For this review, take the finished solid that the model builds, in its own axes (mm). A direction names the side the tool comes from. Round coordinates to 2 decimals unless told otherwise and drop trailing zeros. One line per question, with ' | ' between items.
```python
from build123d import *

# Parameters (mm, degrees)
EXTRUDE_1_DEPTH = 10
SHELL_2_T       = 3
FILLET_3_R      = 10
FILLET_4_R      = 3
SKETCH_2_R      = 2.65
EXTRUDE_2_DEPTH = 8
FILLET_7_R      = 5
CHAMFER_1_SIZE  = 0.2
CHAMFER_2_SIZE  = 0.2
FILLET_9_R      = 2
FILLET_10_R     = 2


# Some blends are built 0.0001 mm under size
with BuildPart() as part:
    # 草图1 → 凸台-拉伸1 (new body)
    with BuildSketch(Plane(origin=(0, 0, 0), x_dir=(1, 0, 0), z_dir=(0, 1, 0))):
        with BuildLine():
            Line((-37.5, 15), (37.5, 15))
            ThreePointArc((37.5, 15), (44.571067812, 12.071067812), (47.5, 5))
            Line((47.5, 5), (47.5, -5))
            ThreePointArc((47.5, -5), (44.571067812, -12.071067812), (37.5, -15))
            Line((37.5, -15), (-37.5, -15))
            ThreePointArc((-37.5, -15), (-44.571067812, -12.071067812), (-47.5, -5))
            Line((-47.5, -5), (-47.5, 5))
            ThreePointArc((-47.5, 5), (-44.571067812, 12.071067812), (-37.5, 15))
        make_face()
    extrude(amount=EXTRUDE_1_DEPTH)

    # 抽壳2
    shell_2_openings = [part.faces().sort_by_distance(p)[0] for p in [
        (0, 0, 0),
    ]]
    offset(amount=SHELL_2_T, openings=shell_2_openings, kind=Kind.INTERSECTION)

    # 圆角3
    # the kernel refuses this fillet: 10 mm, written as the material it takes off along each edge
    with BuildSketch(Plane(origin=(37.5, 13, 5), x_dir=(1, 0, 0), z_dir=(0, 0, -1))) as fillet_3_piece_1:
        with BuildLine():
            CenterArc((13 - FILLET_3_R, FILLET_3_R), FILLET_3_R, 270, 90)
            Line((13 - FILLET_3_R, 0), (13, 0))
            Line((13, 0), (13, FILLET_3_R))
        make_face()
    revolve(axis=Axis((37.5, 13, 5), (0, -1, 0)), revolution_arc=90, mode=Mode.SUBTRACT)
    with BuildSketch(Plane(origin=(50.5, 13, 5), x_dir=(0, -1, 0), z_dir=(0, 0, -1)), Plane(origin=(-50.5, 13, -5), x_dir=(0, -1, 0), z_dir=(0, 0, 1))) as fillet_3_piece_2:
        with BuildLine():
            CenterArc((FILLET_3_R, FILLET_3_R), FILLET_3_R, 180, 90)
            Line((0, FILLET_3_R), (0, 0))
            Line((0, 0), (FILLET_3_R, 0))
        make_face()
    extrude(amount=10, mode=Mode.SUBTRACT)
    with BuildSketch(Plane(origin=(37.5, 13, -5), x_dir=(0, 0, -1), z_dir=(-1, 0, 0))) as fillet_3_piece_3:
        with BuildLine():
            CenterArc((13 - FILLET_3_R, FILLET_3_R), FILLET_3_R, 270, 90)
            Line((13 - FILLET_3_R, 0), (13, 0))
            Line((13, 0), (13, FILLET_3_R))
        make_face()
    revolve(axis=Axis((37.5, 13, -5), (0, -1, 0)), revolution_arc=90, mode=Mode.SUBTRACT)
    with BuildSketch(Plane(origin=(37.5, 13, -18), x_dir=(0, -1, 0), z_dir=(-1, 0, 0)), Plane(origin=(-37.5, 13, 18), x_dir=(0, -1, 0), z_dir=(1, 0, 0))) as fillet_3_piece_4:
        with BuildLine():
            CenterArc((FILLET_3_R, FILLET_3_R), FILLET_3_R, 180, 90)
            Line((0, FILLET_3_R), (0, 0))
            Line((0, 0), (FILLET_3_R, 0))
        make_face()
    extrude(amount=75, mode=Mode.SUBTRACT)
    with BuildSketch(Plane(origin=(-37.5, 13, -5), x_dir=(-1, 0, 0), z_dir=(0, 0, 1))) as fillet_3_piece_5:
        with BuildLine():
            CenterArc((13 - FILLET_3_R, FILLET_3_R), FILLET_3_R, 270, 90)
            Line((13 - FILLET_3_R, 0), (13, 0))
            Line((13, 0), (13, FILLET_3_R))
        make_face()
    revolve(axis=Axis((-37.5, 13, -5), (0, -1, 0)), revolution_arc=90, mode=Mode.SUBTRACT)
    with BuildSketch(Plane(origin=(-37.5, 13, 5), x_dir=(0, 0, 1), z_dir=(1, 0, 0))) as fillet_3_piece_6:
        with BuildLine():
            CenterArc((13 - FILLET_3_R, FILLET_3_R), FILLET_3_R, 270, 90)
            Line((13 - FILLET_3_R, 0), (13, 0))
            Line((13, 0), (13, FILLET_3_R))
        make_face()
    revolve(axis=Axis((-37.5, 13, 5), (0, -1, 0)), revolution_arc=90, mode=Mode.SUBTRACT)

    # 圆角4
    fillet_4_edges = [part.edges().sort_by_distance(p)[0] for p in [
        (50.5, 0, 0),
        (46.692388155, 0, 14.192388155),
        (0, 0, 18),
        (-46.692388155, 0, 14.192388155),
        (-50.5, 0, 0),
        (-46.692388155, 0, -14.192388155),
        (0, 0, -18),
        (46.692388155, 0, -14.192388155),
    ]]
    fillet(fillet_4_edges, radius=FILLET_4_R - 0.0001)  # a hair under: the kernel refuses the full size

    # 草图2 → 凸台-拉伸2 (add)
    # profile 1 of 2: a face of its own
    with BuildSketch(Plane(origin=(0, 10, 0), x_dir=(-1, 0, 0), z_dir=(0, -1, 0))):
        with Locations(Location((36.6, 0, 0), (0, 0, 270))):
            Circle(SKETCH_2_R)
        Polygon((34.55, -0.55), (34.55, 0.55), (36.05, 0.55), (36.05, 2.05), (37.15, 2.05), (37.15, 0.55), (38.65, 0.55), (38.65, -0.55), (37.15, -0.55), (37.15, -2.05), (36.05, -2.05), (36.05, -0.55), align=None, mode=Mode.SUBTRACT)
    # profile 2 of 2: a face of its own
    with BuildSketch(Plane(origin=(0, 10, 0), x_dir=(-1, 0, 0), z_dir=(0, -1, 0))):
        with Locations(Location((-36.6, 0, 0), (0, 0, 90))):
            Circle(SKETCH_2_R)
        Polygon((-37.15, 0.55), (-37.15, 2.05), (-36.05, 2.05), (-36.05, 0.55), (-34.55, 0.55), (-34.55, -0.55), (-36.05, -0.55), (-36.05, -2.05), (-37.15, -2.05), (-37.15, -0.55), (-38.65, -0.55), (-38.65, 0.55), align=None, mode=Mode.SUBTRACT)
    extrude(amount=EXTRUDE_2_DEPTH)

    # 圆角7
    fillet_7_edges = [part.edges().sort_by_distance(p)[0] for p in [
        (-44.571067812, 10, 12.071067812),
        (0, 10, 15),
        (44.571067812, 10, 12.071067812),
        (47.5, 10, 0),
        (44.571067812, 10, -12.071067812),
        (0, 10, -15),
        (-44.571067812, 10, -12.071067812),
        (-47.5, 10, 0),
    ]]
    fillet(fillet_7_edges, radius=FILLET_7_R)

    # 倒角1
    chamfer_1_edges = [part.edges().sort_by_distance(p)[0] for p in [
        (35.3, 2, -0.55),
        (37.15, 2, 1.3),
        (38.65, 2, 0),
        (37.9, 2, -0.55),
        (37.15, 2, -1.3),
        (36.6, 2, -2.05),
        (34.55, 2, 0),
        (35.3, 2, 0.55),
        (36.05, 2, 1.3),
        (36.6, 2, 2.05),
        (37.9, 2, 0.55),
        (36.05, 2, -1.3),
    ]]
    chamfer(chamfer_1_edges, length=CHAMFER_1_SIZE)

    # 倒角2
    chamfer_2_edges = [part.edges().sort_by_distance(p)[0] for p in [
        (-36.6, 2, -2.05),
        (-37.15, 2, -1.3),
        (-37.9, 2, -0.55),
        (-38.65, 2, 0),
        (-37.15, 2, 1.3),
        (-35.3, 2, -0.55),
        (-37.9, 2, 0.55),
        (-36.6, 2, 2.05),
        (-36.05, 2, 1.3),
        (-35.3, 2, 0.55),
        (-34.55, 2, 0),
        (-36.05, 2, -1.3),
    ]]
    chamfer(chamfer_2_edges, length=CHAMFER_2_SIZE)

    # 圆角9
    fillet_9_edges = [part.edges().sort_by_distance(p)[0] for p in [
        (36.6, 10, 2.65),
    ]]
    fillet(fillet_9_edges, radius=FILLET_9_R)

    # 圆角10
    fillet_10_edges = [part.edges().sort_by_distance(p)[0] for p in [
        (-36.6, 10, -2.65),
    ]]
    fillet(fillet_10_edges, radius=FILLET_10_R)


solid = part.part
```
(1) For probe 1 along Z at (x, y) = (34, 9.25); probe 2 along X at (y, z) = (9, -9.5); probe 3 along Z at (x, y) = (38, 6.75), list the stretches that pass through material, from the lowest coordinate up. Write a range as [from, to].
Output values:
probe 1: [-15.81, -12.63], [-1.67, 1.67], [12.63, 15.81] | probe 2: [-47.54, -44.11], [44.11, 47.54] | probe 3: [-17.26, -14.67], [-2.25, -0.55], [0.55, 2.25], [14.67, 17.26]
(2) For faces 5 (the flat face through (1, 13, 0)), 6 (the flat face through (-47.5, 2, 0)), list the 3-axis set-ups (+Z, -Z, +X, -X, +Y, -Y) from which the entire face can be reached by the end or side of a thin tool; tool diameter is ignored.
Output values:
face 5: +Z, -Z, +X, -X, +Y | face 6: -Y
(3) Mouldability with a two-part tool opening along X and no side actions: class faces 1 (the cylindrical face through (47.49, 10.15, 0.07)), 2 (the flat face through (37, 10, 0)), 3 (the cylindrical face through (-47.49, 10.15, -0.07)), 4 (the cylindrical face through (-0.52, 0.86, 17.1)) as released by +X, released by -X, zero draft, split by the parting line, or undercut.
Output values:
face 1: released by +X | face 2: undercut | face 3: released by -X | face 4: zero draft
(4) Insertion check: pin 1 (2 mm diameter, centred on y = 3.5, z = 1, fed in from -X); pin 2 (1.6 mm diameter, centred on y = 7.5, z = -1.5, fed in from +X); pin 3 (1.2 mm diameter, centred on x = 36.5, y = 7, fed in from +Z); pin 4 (0.7 mm diameter, centred on y = 7, z = 1.5, fed in from -X). Each pin has a flat end and moves straight along its axis. Give the tip position at first contact, or say it passes through.
Output values:
pin 1: x = -50.5 | pin 2: x = 49.79 | pin 3: z = 17.4 | pin 4: x = -49.81
